The model under review builds one solid part; all positions refer to its coordinate system, in mm. Face numbers are marked on the shaded views. A direction names the side the tool comes from. Coordinates: 2 decimals unless noted, no trailing zeros. Loops run counter-clockwise (first coordinate to the right, second up) from the corner with the lowest first, then second, coordinate; pieces in that order, holes last. Notation, with made-up numbers: M 12,52.5 L 27,52.5 A15 ccw 27,59.5 Z; hole C -7.5,-20.75 d4. An arc over 180 degrees is marked long. Write item = value, one per line. Start each with the question number.
Q1. Mouldability with a two-part tool opening along X and no side actions: class the marked faces 3, 4 and 5 as released by +X, released by -X, zero draft, split by the parting line, or undercut.
Q2. For the marked faces 1 and 2, list the 3-axis set-ups (+Z, -Z, +X, -X, +Y, -Y) from which the entire face can be reached by the end or side of a thin tool; tool diameter is ignored.
Q3. Clearance check with flat-ended pins moving along their axes: pin 1 Ø21.5 at (y, z) = (81, -0.5) entering from -X; pin 2 Ø1.5 at (x, y) = (36, 84.5) entering from -Z; pin 3 Ø4 at (x, y) = (7, 16.5) entering from -Z; pin 4 Ø10 at (x, y) = (25, 47) entering from +Z. State where each tip first meets the part, or that it passes through.
Q4. We need section A-A on z = 0. Give the boundary of the cut face in (x, y), and give its area (3 significant figures).
Q5. Wall thickness on probe 1 along Z at (x, y) = (0, 12); probe 2 along X at (y, z) = (54.5, 8); probe 3 along Y at (x, z) = (42, 0): over which ranges is each line inside the solid? List them lowest first.
Q6. We need section B-B on y = 16.5. Give the boundary of the cut face in (x, z), and give its area (3 significant figures).
Autodesk Inventor part; units mm, degrees
ref_plane "YZ Plane" through (0, 0, 0) normal (1, 0, 0) x (0, 1, 0)
ref_plane "XZ Plane" through (0, 0, 0) normal (0, 1, 0) x (-1, 0, 0)
ref_plane "XY Plane" through (0, 0, 0) normal (0, 0, 1) x (1, 0, 0)
sketch "Sketch1" plane through (0, 0, 0) normal (0, 0, 1) x (1, 0, 0)
  line L0 (0, 0) -> (0, 38.1)
  line L1 (38.1, 76.2) -> (50.8, 76.2)
  arc A0 (38.1, 76.2) -> (0, 38.1) centre (38.1, 38.1) ccw
  dimension "d1" = 76.2
  dimension "d2" = 50.8
  dimension "d4" = 38.1
sketch "Sketch2" plane through (0, 0, 0) normal (0, 1, 0) x (-1, 0, 0)
  circle A0 centre (0, 0) radius 12.7
  circle A1 centre (0, 0) radius 11.05
  dimension "d3" = 25.4
  dimension "d11" = 1.65
sweep "Sweep1" add profiles "Sketch2" path "Sketch1"
sketch "Sketch3" plane through (50.8, 76.2, 0) normal (1, 0, 0) x (0, 0, -1)
  circle A0 centre (0, 0) radius 12.7
  circle A1 centre (0, 0) radius 25.15
  point P0 (0, -76.2)
  dimension "d6" = 50.3
extrude "Extrusion1" add sketch "Sketch3" against normal blind 5
chamfer "Chamfer1" distance 3 distance2 3.8692 1 edges at (45.8, 76.2, 25.15) measured on face at (47.4667, 72.1657, -24.8243)
equation "\"d4\" = 0.75 * d2"
equation "\"d15\" = 0.0769231 * d6"
properties part number "Ferrule 90 deg Elb-25.4"
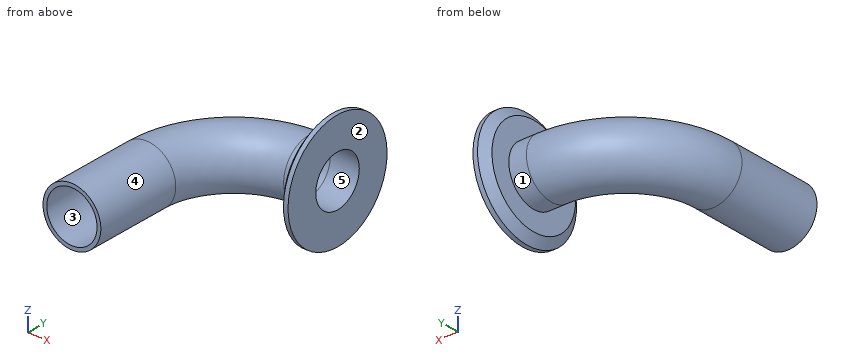
Returned:
q1.face_3 = undercut
q1.face_4 = split by the parting line
q1.face_5 = zero draft
q2.face_1 = none
q2.face_2 = +Z, -Z, +X, +Y, -Y
q3.pin_1 = -1.23
q3.pin_2 = -10.18
q3.pin_3 = -11.67
q3.pin_4 = through
q4.outline = M -12.7,0 L -11.05,0 L -11.05,38.1 A49.15 cw 38.1,87.25 L 50.8,87.25 L 50.8,101.35 L 48.8,101.35 L 45.8,97.48 L 45.8,88.9 L 38.1,88.9 A50.8 ccw -12.7,38.1 Z; M 11.05,0 L 12.7,0 L 12.7,38.1 A25.4 cw 38.1,63.5 L 45.8,63.5 L 45.8,54.92 L 48.8,51.05 L 50.8,51.05 L 50.8,65.15 L 38.1,65.15 A27.05 ccw 11.05,38.1 Z
q4.area = 478 mm^2
q5.probe_1 = -12.7 to -11.05, 11.05 to 12.7
q5.probe_2 = -6.97 to -4.58, 12.41 to 15.11, 47.23 to 50.8
q5.probe_3 = 63.5 to 65.15, 87.25 to 88.9
q6.outline = C 0,0 d25.4; hole C 0,0 d22.1
q6.area = 123 mm^2
